Can you work these out from the model? Positions are in its coordinate system, mm. A direction names the side the tool comes from. Give positions to 0.01 mm unless a question says otherwise; leave off trailing zeros. Write each loop counter-clockwise with the first axis right and the second up, starting at its lowest first coordinate (ties: lowest second). Pieces come first, ordered by that corner, then holes.
```python
from build123d import *

# Parameters (mm, degrees)
F1_DEPTH  = 56
F3_DEPTH  = 116
F5_D      = 12
F5_DEPTH  = 5
F5_TIP    = 3.6051637142
F7_D      = 4
F7_DEPTH  = 6
F7_TIP    = 1.2017212381
F9_D      = 4
F9_DEPTH  = 6
F9_TIP    = 1.2017212381
F11_DEPTH = 56.001
F13_D     = 3
F13_DEPTH = 4
F13_TIP   = 0.9012909285


# Not quite as in the source:
# - a feature names something its author has since deleted; it is built from what else it names


with BuildPart() as f1:
    # F0 (on Front) → F1 (new body)
    with BuildSketch(Plane.XZ):
        Polygon((1.5, 0), (2, 2), (12, 2), (12.5, 0), (58, 0), (58, 20), (-58, 20), (-58, 0), (-12.5, 0), (-12, 2), (-2, 2), (-1.5, 0), (0, 0), align=None)
    extrude(amount=F1_DEPTH)

    # F2 (on face) → F3 (cut, through all)
    with BuildSketch(Plane(origin=(-58, 0, 0), x_dir=(0, -1, 0), z_dir=(-1, 0, 0))):
        Polygon((28, 20), (20.0020753821, 20), (13, 10), (28, 10), align=None)
        Polygon((35.9979246179, 20), (28, 20), (28, 10), (43, 10), align=None)
    extrude(amount=-F3_DEPTH, mode=Mode.SUBTRACT)

    # F5
    with Locations(Plane.XY.offset(10)):
        with Locations((0, -28)):
            Hole(F5_D / 2, depth=F5_DEPTH)
            with Locations((0, 0, -(F5_DEPTH + F5_TIP / 2))):  # 118° drill point
                Cone(0, F5_D / 2, F5_TIP, mode=Mode.SUBTRACT)

    # F7
    with Locations(Plane(origin=(-58, 0, 0), x_dir=(0, -1, 0), z_dir=(-1, 0, 0))):
        with Locations((28, 5)):
            Hole(F7_D / 2, depth=F7_DEPTH)
            with Locations((0, 0, -(F7_DEPTH + F7_TIP / 2))):  # 118° drill point
                Cone(0, F7_D / 2, F7_TIP, mode=Mode.SUBTRACT)

    # F9
    with Locations(Plane.YZ.offset(58)):
        with Locations((-28, 5)):
            Hole(F9_D / 2, depth=F9_DEPTH)
            with Locations((0, 0, -(F9_DEPTH + F9_TIP / 2))):  # 118° drill point
                Cone(0, F9_D / 2, F9_TIP, mode=Mode.SUBTRACT)

    # F10 (on face) → F11 (cut, through all)
    with BuildSketch(Plane.XZ.offset(56)):
        Polygon((12.5, 0), (20, 0), (20, 3), (28, 3), (28, 5), (20, 5), (0, 5), (0, 0), (1.5, 0), (2, 2), (12, 2), align=None)
        Polygon((-1.5, 0), (0, 0), (0, 5), (-20, 5), (-28, 5), (-28, 3), (-20, 3), (-20, 0), (-12.5, 0), (-12, 2), (-2, 2), align=None)
    extrude(amount=-F11_DEPTH, mode=Mode.SUBTRACT)

    # F13
    with Locations(Plane(origin=(0, 0, 0), x_dir=(1, 0, 0), z_dir=(0, 0, -1))):
        with Locations((-24, 46), (24, 46), (24, 10), (-24, 10)):
            Hole(F13_D / 2, depth=F13_DEPTH)
            with Locations((0, 0, -(F13_DEPTH + F13_TIP / 2))):  # 118° drill point
                Cone(0, F13_D / 2, F13_TIP, mode=Mode.SUBTRACT)


solid = f1.part
```
1) Suppose I cut it at D-D on x = -39.5. Write out the boundary of the cut face in (y, z).
Values follow:
outline: (-56, 0) - (0, 0) - (0, 20) - (-20, 20) - (-13, 10) - (-43, 10) - (-36, 20) - (-56, 20) - close
2) For faces 5 (the face through (54.958, -29.908, 5.601)), 6 (the face through (24.325, -44.536, 1.521)), 7 (the face through (-28, -28, 4)), 8 (the face through (-0.81, -16.55, 15.07)), which set-ups out of +Z, -Z, +X, -X, +Y, -Y let a thin tool reach every point of the face, with its end or its side?
Values follow:
face 5: +X
face 6: -Z
face 7: +Y, -Y
face 8: +X, -X
3) If we mould it in two halves opening along Y, with no side actions, what happens to faces 1 (the face through (0, -35, 5)), 2 (the face through (1.301, -33.857, 7.465)), 3 (the face through (-1, -56, 10)), 4 (the face through (-22.5, -10.07, 1.52))? For each: +Y half, -Y half, draft (parallel to the pull), parting line (faces both ways), or undercut.
Values follow:
face 1: draft
face 2: undercut
face 3: -Y half
face 4: undercut
4) Suppose I cut it at B-B on y = -46. Write out the boundary of the cut face in (x, z).
Values follow:
outline: (-58, 0) - (-25.5, 0) - (-25.5, 3) - (-28, 3) - (-28, 5) - (28, 5) - (28, 3) - (25.5, 3) - (25.5, 0) - (58, 0) - (58, 20) - (-58, 20) - close; (-22.5, 0) - (-20, 0) - (-20, 3) - (-22.5, 3) - close; (20, 0) - (22.5, 0) - (22.5, 3) - (20, 3) - close
5) Suppose I cut it at C-C on z = 16.25. Write out the boundary of the cut face in (x, y), plus the area to 3 significant figures.
Values follow:
outline: (-58, -56) - (58, -56) - (58, -38.62) - (-58, -38.62) - close; (-58, -17.38) - (58, -17.38) - (58, 0) - (-58, 0) - close
area: 4,030 mm2
6) Suppose I cut it at A-A on x = 0. Write out the boundary of the cut face in (y, z).
Values follow:
outline: (-56, 5) - (-34, 5) - (-34, 10) - (-43, 10) - (-36, 20) - (-56, 20) - close; (-22, 5) - (0, 5) - (0, 20) - (-20, 20) - (-13, 10) - (-22, 10) - close
7) Please list where these lines run through material, in increasing order: L1, parallel to Y at x = 24, z = 2.05; L2, parallel to X at y = -46, z = 2.1; L3, parallel to Z at x = 55.9, y = -28.
Values follow:
L1: y = -56 to -47.5, -44.5 to -11.5, -8.5 to 0
L2: x = -58 to -25.5, -22.5 to -20, 20 to 22.5, 25.5 to 58
L3: z = 0 to 3, 7 to 10
8) For pin 1 Ø12 at (x, z) = (37.5, 11.5) entering from +Y; pin 2 Ø19 at (x, y) = (0, -28) entering from -Z; pin 3 Ø3.5 at (y, z) = (-28, 5) entering from -X, each with a flat end and sliding along its axis, tell me the tip position at first contact or that it passes through.
Values follow:
pin 1: stops at y = 0
pin 2: stops at z = 5
pin 3: stops at x = -51.85
